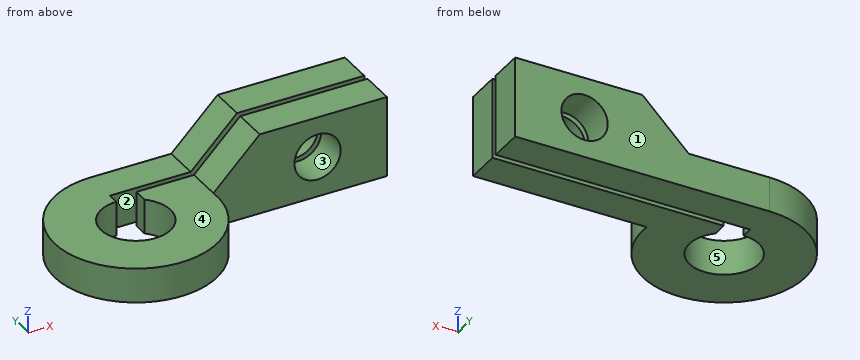
```python
from build123d import *

# Parameters (mm, degrees)
F1_DEPTH = 3
F2_W     = 15
F2_H     = 3
F3_DEPTH = 4
F5_DEPTH = 6.501
F6_R     = 2
F7_DEPTH = 6.501


with BuildPart() as f1:
    # F0 (on Top) → F1 (new body)
    with BuildSketch(Plane.XY):
        with BuildLine():
            ThreePointArc((2, 2.236068), (-1.070466, -2.802517), (0, 3))
            Line((0, 3), (0, 4))
            Line((0, 4), (21.98212, 4))
            Line((21.98212, 4), (21.98212, 7))
            Line((21.98212, 7), (0, 7))
            ThreePointArc((0, 7), (-4.769696, -5.123475), (6.98212, 0.5))
            Line((6.98212, 0.5), (21.98212, 0.5))
            Line((21.98212, 0.5), (21.98212, 3.5))
            Line((21.98212, 3.5), (2, 3.5))
            Line((2, 3.5), (2, 2.236068))
        make_face()
    extrude(amount=F1_DEPTH)

    # F2 (on face) → F3 (join)
    with BuildSketch(Plane.XY.offset(3)):
        with Locations((14.48212, 5.5)):
            Rectangle(F2_W, F2_H)
        with Locations((14.48212, 2)):
            Rectangle(F2_W, F2_H)
    extrude(amount=F3_DEPTH)

    # F4 (on face) → F5 (cut, through all)
    with BuildSketch(Plane.XZ.offset(-0.5)):
        Polygon((6.98212, 7), (6.98212, 3), (10.98212, 7), align=None)
    extrude(amount=-F5_DEPTH, mode=Mode.SUBTRACT)

    # F6 (on face) → F7 (cut, through all)
    with BuildSketch(Plane.XZ.offset(-0.5)):
        with Locations((15.98212, 3.5)):
            Circle(F6_R)
    extrude(amount=-F7_DEPTH, mode=Mode.SUBTRACT)


solid = f1.part
```
Geometry: final body of the model. Coordinates: model frame, mm. Face numbers are marked on the shaded views. A direction names the side the tool comes from. Give positions to 0.01 mm unless a question says otherwise; leave off trailing zeros. Loops run counter-clockwise (first coordinate to the right, second up) from the corner with the lowest first, then second, coordinate; pieces in that order, holes last. Notation, with made-up numbers: (31.5, 57.5) -> (68.5, 57.5) arc R20 ccw to (68.5, 86.5) -> close; hole circle Ø6 at (30.5, 50). An arc over 180 degrees is marked (long way). Use CSV: the item, a comma, the result in double quotes.
(1) Ray query, line 1 along X through (y, z) = (0, 2.1); line 2 along Y through (x, z) = (17, 5.75); line 3 along Y through (x, z) = (-0.5, 0.5). Return the intervals inside material, ascending. Write a range as [from, to].
From the geometry:
line 1,"[-7, -3], [3, 7]"
line 2,"[0.5, 3.5], [4, 7]"
line 3,"[-6.98, -2.96], [2.96, 6.98]"
(2) Cut plane D-D (y = 4.75). Output: boundary loops of the cut face in (x, z).
From the geometry:
outline,"(-5.14, 0) -> (21.98, 0) -> (21.98, 7) -> (10.98, 7) -> (6.98, 3) -> (-5.14, 3) -> close; hole circle Ø4 at (15.98, 3.5)"
(3) Access query for the marked faces 4 and 5. Directions: +Z, -Z, +X, -X, +Y, -Y. A direction counts if a zero-diameter tool reaches every point of the face in a straight line with its end or side. Return the directions, or none.
From the geometry:
face 4,"+Z, -X, +Y, -Y"
face 5,"+Z, -Z"
(4) Cut plane C-C (x = 1.5). Output: boundary loops of the cut face in (y, z).
From the geometry:
outline,"(-6.84, 0) -> (-2.6, 0) -> (-2.6, 3) -> (-6.84, 3) -> close; (4, 0) -> (7, 0) -> (7, 3) -> (4, 3) -> close"
(5) Cut plane B-B (z = 4.5). Output: boundary loops of the cut face in (x, y).
From the geometry:
outline,"(8.48, 0.5) -> (14.25, 0.5) -> (14.25, 3.5) -> (8.48, 3.5) -> close; (8.48, 4) -> (14.25, 4) -> (14.25, 7) -> (8.48, 7) -> close; (17.71, 0.5) -> (21.98, 0.5) -> (21.98, 3.5) -> (17.71, 3.5) -> close; (17.71, 4) -> (21.98, 4) -> (21.98, 7) -> (17.71, 7) -> close"
(6) Cut plane A-A (y = 0). Output: boundary loops of the cut face in (x, z), plus the area to 3 significant figures.
From the geometry:
outline,"(-7, 0) -> (-3, 0) -> (-3, 3) -> (-7, 3) -> close; (3, 0) -> (7, 0) -> (7, 3) -> (3, 3) -> close"
area,"24.0 mm^2"
(7) First-contact query: P1, Ø2.5, axis at x = 15.98, z = 3.5, coming from the +Y side; P2, Ø4, axis at x = 3, y = 0, coming from the +Z side; P3, Ø3, axis at x = -3, z = 3, coming from the +Y side; P4, Ø5, axis at x = 6.5, y = 3, coming from the +Z side. Flat tips, straight axial feed; report the tip coordinate or a pass-through.
From the geometry:
P1,"through"
P2,"z = 3"
P3,"y = 6.84"
P4,"z = 5.02"
(8) Pull-direction query (Y, two-part tool) for the marked faces 1, 2 and 3; classes: released by +Y, released by -Y, zero draft, split by the parting line, or undercut.
From the geometry:
face 1,"released by +Y"
face 2,"undercut"
face 3,"zero draft"
